Verification items for the finished model (mm, model axes). Give positions to 0.01 mm unless a question says otherwise; leave off trailing zeros. Order: outer loops, then holes, each group sorted by start corner. A loop starts at its lowest first (then second) coordinate and runs counter-clockwise, first axis right, second up. Notation, with made-up numbers: (-24.5, -23.75) - (19.5, -23.75) arc R22 cw to (19.5, -7.75) - close; hole circle Ø1 at (34.25, 81.25). An arc over 180 degrees is marked (long way). Answer as a JSON object with one key per item and string values.
```python
from build123d import *

# Parameters (mm, degrees)
SKETCH1_R           = 4.7625
BOSS_EXTRUDE1_DEPTH = 44.45
CHAMFER1_SIZE       = 1.524


with BuildPart() as part:
    # Sketch1 → Boss-Extrude1 (new body)
    with BuildSketch(Plane.XY):
        Circle(SKETCH1_R)
    extrude(amount=-BOSS_EXTRUDE1_DEPTH)

    # Sketch2 → Cut-Revolve1 (revolve, cut)
    with BuildSketch(Plane(origin=(0, 0, 0), x_dir=(1, 0, 0), z_dir=(0, 1, 0)), mode=Mode.PRIVATE) as cut_revolve1_sk:
        Polygon((-4.7625, 33.655), (-4.7625, 32.4866), (-4.4831, 32.4866), (-4.4831, 33.420555563), align=None)
    revolve(cut_revolve1_sk.sketch.rotate(Axis((0, 0, -44.45), (0, 0, 1)), 180), axis=Axis((0, 0, -44.45), (0, 0, 1)), mode=Mode.SUBTRACT)

    # Chamfer1
    chamfer1_edges = [part.edges().sort_by_distance(p)[0] for p in [
        (-4.7625, 0, 0),
        (-4.7625, 0, -44.45),
    ]]
    chamfer(chamfer1_edges, length=CHAMFER1_SIZE)


solid = part.part
```
(1) Section check A-A (z = -3). Record the cut outline in (x, y) (1 decimal), then the cut area to 3 significant figures.
Computed values:
{"outline": "circle Ø9.5 at (0, 0)", "area": "71.3 mm²"}
(2) Material ranges on line 1 along Y through (x, z) = (-0.25, -36); line 2 along Z through (x, y) = (-2.75, -3.75); line 3 along Z through (x, y) = (-1.5, 4), recorded low to high. Write a range as [from, to].
Computed values:
{"line 1": "y = [-4.76, 4.76]", "line 2": "z = [-43.04, -33.56], [-32.49, -1.41]", "line 3": "z = [-43.42, -1.03]"}
(3) Release check for a two-part mould opening along Z. For faces 1 (the flat face through (0, 0, 0)), 2 (the cylindrical face through (-0.972, -4.376, -32.96)), 3 (the flat face through (0, 0, -44.45)), 4 (the cylindrical face through (-3.78, -2.9, -16.79)) record: pulls with the +Z half, pulls with the -Z half, needs draft (parallel to the pull), parting line crosses it, or undercut.
Computed values:
{"face 1": "pulls with the +Z half", "face 2": "undercut", "face 3": "pulls with the -Z half", "face 4": "needs draft"}
(4) Gauge pin test, flat end, axial feed: pin 1 Ø1 at (x, z) = (2, -35.5) entering from +Y. Record the tip position at first contact, or that the pin passes through.
Computed values:
{"pin 1": "stops at y = 4.52"}
